The listing builds one solid part. Answer for the finished solid, in the listing's coordinates (mm). Face numbers are marked on the shaded views. A direction names the side the tool comes from. Round coordinates to 2 decimals unless told otherwise and drop trailing zeros. Write each loop counter-clockwise with the first axis right and the second up, starting at its lowest first coordinate (ties: lowest second). Pieces come first, ordered by that corner, then holes. Notation, with made-up numbers: (37.5, -8) - (70.5, -8) arc R11 ccw to (70.5, 12) - close; hole circle Ø4 at (11, -34). An arc over 180 degrees is marked (long way). Use a Markdown table: item, result. Add a question column.
1) Find the intervals of material crossed by probe 1 along Z at (x, y) = (0, -2.25); probe 2 along Z at (x, y) = (0, -0.25); probe 3 along Y at (x, z) = (-12, 5), in increasing order. Write a range as from..to.
2) A cutting plane is placed at B-B (z = 0). Give the vertices of the cut face in (x, y).
3) A cutting plane is placed at A-A (x = 0). Give the vertices of the cut face in (y, z), then the cut area to 3 significant figures.
4) A cutting plane is placed at C-C (y = -2.5). Give the vertices of the cut face in (x, z), then the cut area to 3 significant figures.
5) Each of these flat-tipped pins is pushed along its axis until it touches: P1, Ø5.5, axis at x = 0, z = 0, coming from the -Y side; P2, Ø2, axis at y = -2.5, z = 2.5, coming from the -X side; P3, Ø1, axis at x = 10.5, y = 0.5, coming from the -Z side; P4, Ø2, axis at x = -9, y = 1, coming from the +Z side. Where does it stop, or does it pass through?
6) A cutting plane is placed at D-D (y = 0.75). Give the vertices of the cut face in (x, z).
7) A tool of negligible diameter and unlimited length cuts with its end or side. For the marked faces 4 and 5, from which of +Z, -Z, +X, -X, +Y, -Y can it reach the whole face along a straight path? Write none if from no direction.
8) Determine the mould class of the marked faces 1, 2 and 3 for opening direction X: +X half, -X half, draft (parallel to the pull), parting line (faces both ways), or undercut.
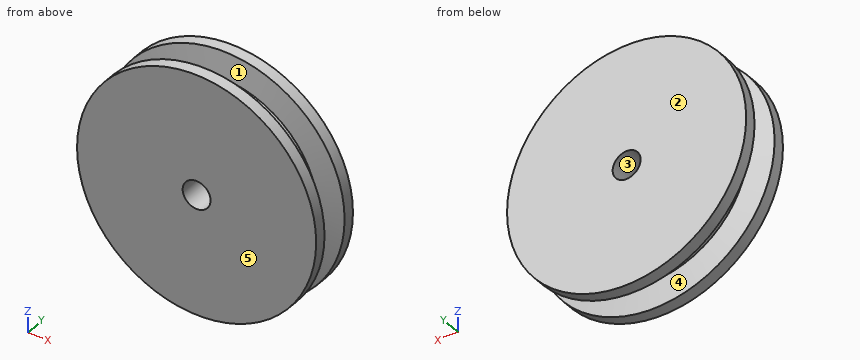
Autodesk Inventor part; units mm, degrees
ref_plane "YZ Plane" through (0, 0, 0) normal (1, 0, 0) x (0, 1, 0)
ref_plane "XZ Plane" through (0, 0, 0) normal (0, 1, 0) x (-1, 0, 0)
ref_plane "XY Plane" through (0, 0, 0) normal (0, 0, 1) x (1, 0, 0)
sketch "스케치1" plane through (0, 0, 0) normal (0, 0, 1) x (1, 0, 0)
  line L0 (0, 0) -> (12, 0) construction
  line L1 (12, 0) -> (12, 1.3)
  line L2 (12, 1.3) -> (15, 1.8)
  line L3 (15, 1.8) -> (15, 3.3)
  line L4 (15, 3.3) -> (0, 3.3)
  line L5 (0, 3.3) -> (0, 0)
  line L6 (12, 0) -> (12, -1.3)
  line L7 (12, -1.3) -> (15, -1.8)
  line L8 (15, -1.8) -> (15, -3.3)
  line L9 (15, -3.3) -> (0, -3.3)
  line L10 (0, -3.3) -> (0, 0)
  line L11 (1.75, 3.3) -> (1.75, -3.3)
  dimension "d0" = 3.3
  dimension "d1" = 15
  dimension "d2" = 12
  dimension "d3" = 0.5
  dimension "d4" = 1.5
  dimension "d6" = 1.75
revolve "회전1" add sketch "스케치1" angle 360 about axis through (0, 3.3, 0) along (0, -1, 0) contours L6 L7 L8 L9 L11 L4 L3 L2 L1
properties part number "회전 축 휠"
Entries:
| question | item | result |
|---|---|---|
| 1 | probe 1 | z = -15..-1.75, 1.75..15 |
| 1 | probe 2 | z = -12..-1.75, 1.75..12 |
| 1 | probe 3 | y = -3.3..-1.47, 1.47..3.3 |
| 2 | outline | (-15, -3.3) - (-1.75, -3.3) - (-1.75, 3.3) - (-15, 3.3) - (-15, 1.8) - (-12, 1.3) - (-12, -1.3) - (-15, -1.8) - close; (1.75, -3.3) - (15, -3.3) - (15, -1.8) - (12, -1.3) - (12, 1.3) - (15, 1.8) - (15, 3.3) - (1.75, 3.3) - close |
| 3 | outline | (-3.3, -15) - (-1.8, -15) - (-1.3, -12) - (1.3, -12) - (1.8, -15) - (3.3, -15) - (3.3, -1.75) - (-3.3, -1.75) - close; (-3.3, 1.75) - (3.3, 1.75) - (3.3, 15) - (1.8, 15) - (1.3, 12) - (-1.3, 12) - (-1.8, 15) - (-3.3, 15) - close |
| 3 | area | 156 mm² |
| 4 | outline | circle Ø30 at (0, 0); hole circle Ø3.5 at (0, 0) |
| 4 | area | 697 mm² |
| 5 | P1 | stops at y = -3.3 |
| 5 | P2 | stops at x = -14.92 |
| 5 | P3 | stops at z = -6.63 |
| 5 | P4 | stops at z = 12.43 |
| 6 | outline | circle Ø24 at (0, 0); hole circle Ø3.5 at (0, 0) |
| 7 | face 4 | none |
| 7 | face 5 | +Z, -Z, +X, -X, -Y |
| 8 | face 1 | parting line |
| 8 | face 2 | draft |
| 8 | face 3 | undercut |
